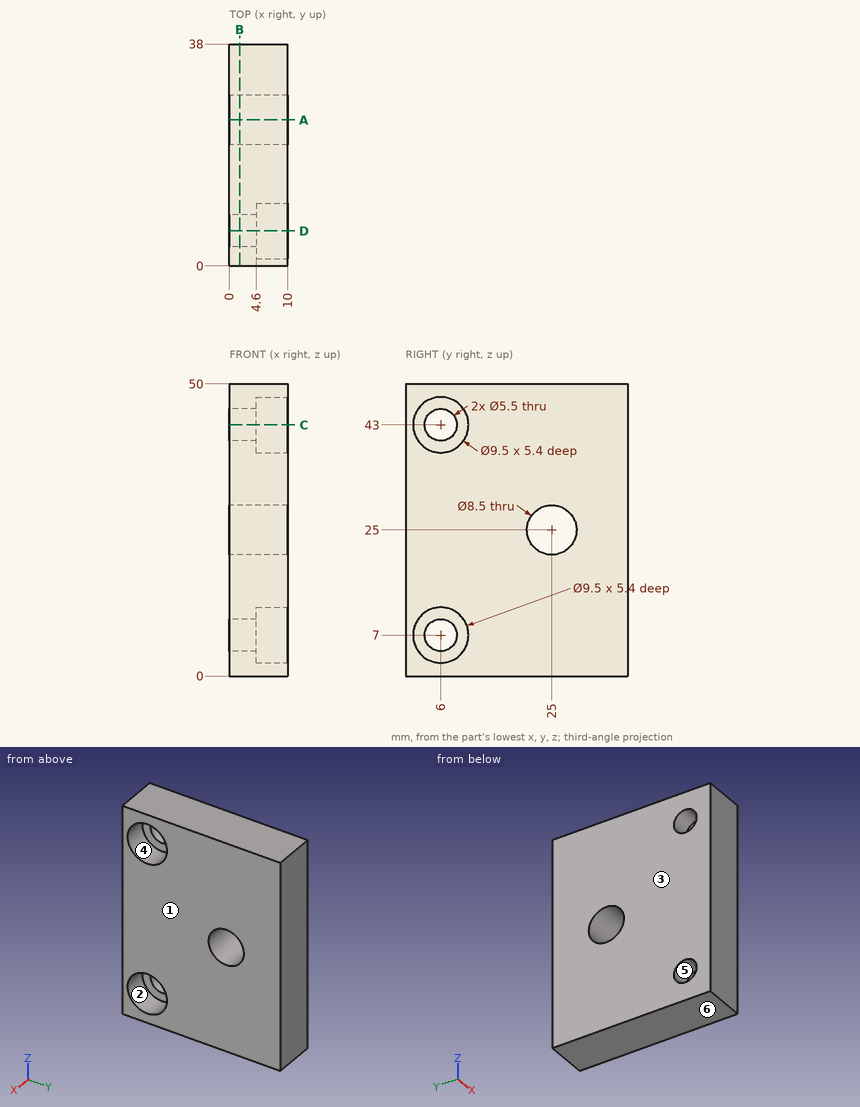
For this review, use the dimensioned drawing (mm, ordinates from the lowest corner) and the shaded views. A direction names the side the tool comes from. Round coordinates to 2 decimals unless told otherwise and drop trailing zeros. Write each loop counter-clockwise with the first axis right and the second up, starting at its lowest first coordinate (ties: lowest second). Pieces come first, ordered by that corner, then holes. Notation, with made-up numbers: (64.25, 9) - (119.25, 9) arc R28 cw to (119.25, 34) - close; hole circle Ø10 at (-23.5, 27). An arc over 180 degrees is marked (long way). Answer as CSV lines item,"result". Start each with the question number.
(1) For the marked faces 1 and 2, list the 3-axis set-ups (+Z, -Z, +X, -X, +Y, -Y) from which the entire face can be reached by the end or side of a thin tool; tool diameter is ignored.
(2) To check wall thickness, follow line 1 (Y direction, x = 6.65, z = 43); line 2 (Y direction, x = 5.75, z = 25); line 3 (Z direction, x = 6, y = 4.5). State the ranges of each line that lie inside material, in increasing order.
(3) We need section B-B on x = 1.75. State the section outline as (y, z) points.
(4) We need section A-A on y = 25. State the section outline as (x, z) points.
(5) Draft analysis for pull direction Z (two halves, no side actions). For the marked faces 3, 4, 5 and 6, state which applies: pulls with the +Z half, pulls with the -Z half, needs draft (parallel to the pull), parting line crosses it, or undercut.
(6) For pin 1 Ø9 at (y, z) = (6, 43) entering from +X, flat-tipped, find the tip position at first contact; note if it passes through.
(7) We need section D-D on y = 6. State the section outline as (x, z) points.
(8) We need section C-C on z = 43. State the section outline as (x, y) points, plus the area to 3 significant figures.
Worked answers:
1,face 1,"+Z, -Z, +X, +Y, -Y"
1,face 2,"+X"
2,line 1,"0 to 1.25, 10.75 to 38"
2,line 2,"0 to 20.75, 29.25 to 38"
2,line 3,"0 to 2.49, 11.51 to 38.49, 47.51 to 50"
3,outline,"(0, 0) - (38, 0) - (38, 50) - (0, 50) - close; hole circle Ø5.5 at (6, 7); hole circle Ø5.5 at (6, 43); hole circle Ø8.5 at (25, 25)"
4,outline,"(0, 0) - (10, 0) - (10, 20.75) - (0, 20.75) - close; (0, 29.25) - (10, 29.25) - (10, 50) - (0, 50) - close"
5,face 3,"needs draft"
5,face 4,"undercut"
5,face 5,"undercut"
5,face 6,"pulls with the -Z half"
6,pin 1,"x = 4.6"
7,outline,"(0, 0) - (10, 0) - (10, 2.25) - (4.6, 2.25) - (4.6, 4.25) - (0, 4.25) - close; (0, 9.75) - (4.6, 9.75) - (4.6, 11.75) - (10, 11.75) - (10, 38.25) - (4.6, 38.25) - (4.6, 40.25) - (0, 40.25) - close; (0, 45.75) - (4.6, 45.75) - (4.6, 47.75) - (10, 47.75) - (10, 50) - (0, 50) - close"
8,outline,"(0, 0) - (10, 0) - (10, 1.25) - (4.6, 1.25) - (4.6, 3.25) - (0, 3.25) - close; (0, 8.75) - (4.6, 8.75) - (4.6, 10.75) - (10, 10.75) - (10, 38) - (0, 38) - close"
8,area,"303 mm²"
